from build123d import *

# Parameters (mm, degrees)
SKETCH1_W           = 190
SKETCH1_H           = 190
BOSS_EXTRUDE1_DEPTH = 5
SKETCH2_W           = 166
SKETCH2_H           = 166
CUT_EXTRUDE1_DEPTH  = 135.443296597
FILLET1_R           = 20
SKETCH3_R           = 3.05
CUT_EXTRUDE2_DEPTH  = 135.443296597
CHAMFER1_SIZE       = 10


with BuildPart() as part:
    # Sketch1 → Boss-Extrude1 (new body)
    with BuildSketch(Plane(origin=(0, 0, 0), x_dir=(1, 0, 0), z_dir=(0, 1, 0))):
        Rectangle(SKETCH1_W, SKETCH1_H)
    extrude(amount=BOSS_EXTRUDE1_DEPTH)

    # Sketch2 → Cut-Extrude1 (cut, through all)
    with BuildSketch(Plane(origin=(0, 5, 0), x_dir=(1, 0, 0), z_dir=(0, 1, 0))):
        Rectangle(SKETCH2_W, SKETCH2_H)
    extrude(amount=-CUT_EXTRUDE1_DEPTH, mode=Mode.SUBTRACT)

    # Fillet1
    fillet1_edges = [part.edges().sort_by_distance(p)[0] for p in [
        (83, 2.5, -83),
        (83, 2.5, 83),
        (-83, 2.5, 83),
        (-83, 2.5, -83),
    ]]
    fillet(fillet1_edges, radius=FILLET1_R)

    # Sketch3 → Cut-Extrude2 (cut, through all)
    with BuildSketch(Plane(origin=(0, 5, 0), x_dir=(1, 0, 0), z_dir=(0, 1, 0))):
        with Locations(Location((-77, 89, 0), (0, 0, 270))):
            Circle(SKETCH3_R)
        with Locations(Location((-89, 68, 0), (0, 0, 270))):
            Circle(SKETCH3_R)
        with Locations(Location((89, 77, 0), (0, 0, 270))):
            Circle(SKETCH3_R)
        with Locations(Location((68, 89, 0), (0, 0, 270))):
            Circle(SKETCH3_R)
        with Locations(Location((77, -89, 0), (0, 0, 270))):
            Circle(SKETCH3_R)
        with Locations(Location((89, -68, 0), (0, 0, 270))):
            Circle(SKETCH3_R)
        with Locations(Location((-89, -77, 0), (0, 0, 270))):
            Circle(SKETCH3_R)
        with Locations(Location((-68, -89, 0), (0, 0, 270))):
            Circle(SKETCH3_R)
    extrude(amount=-CUT_EXTRUDE2_DEPTH, mode=Mode.SUBTRACT)

    # Chamfer1
    chamfer1_edges = [part.edges().sort_by_distance(p)[0] for p in [
        (-95, 2.5, -95),
        (-95, 2.5, 95),
        (95, 2.5, 95),
        (95, 2.5, -95),
    ]]
    chamfer(chamfer1_edges, length=CHAMFER1_SIZE)


solid = part.part
Geometry: final body of the model. Coordinates: model frame, mm. A direction names the side the tool comes from. Round coordinates to 2 decimals unless told otherwise and drop trailing zeros. Loops run counter-clockwise (first coordinate to the right, second up) from the corner with the lowest first, then second, coordinate; pieces in that order, holes last. Notation, with made-up numbers: (-29, 17) -> (9, 17) arc R25 ccw to (9, 49) -> close; hole circle Ø2 at (24, -14). An arc over 180 degrees is marked (long way). One line per question, with ' | ' between items. Start each with the question number.
1. Mould query, pull axis X, two halves, no side actions, for faces 1 (the face through (90, 2, 90)), 2 (the face through (-86, 0, -1)), 3 (the face through (-95, 2, 1)), 4 (the face through (-88.866, 2.535, 73.953)). Classes: pulls with the +X half, pulls with the -X half, needs draft (parallel to the pull), parting line crosses it, or undercut.
2. Line query: line 1 along X through (y, z) = (3.05, -52); line 2 along X through (y, z) = (1.7, 68); line 3 along X through (y, z) = (2.25, 89). Output: solid intervals per line, ascending. Write a range as [from, to].
3. Section A-A on z = 49. Output: boundary loops of the cut face in (x, y), and give its area (3 significant figures).
4. Section D-D on y = 1.85. Count the separate pieces of the cut face and the enclosed holes in it, and give its area (3 significant figures).
5. Section C-C on x = 89. Output: boundary loops of the cut face in (y, z).
6. Section B-B on x = -48. Output: boundary loops of the cut face in (y, z), and give its area (3 significant figures).
7. Set-up query: faces 5 (the face through (-83, 3, 1)), 6 (the face through (95, 2, 1)). Return all of +Z, -Z, +X, -X, +Y, -Y with unobstructed straight access to the full face (end or side cutting, diameter ignored); none if empty.
8. Contact query for a flat-ended pin moving along its axis: pin 1 (3.5 mm diameter, centred on x = 89, z = -77, fed in from +Y). Output: stop coordinate, or through.
Returned:
1) face 1: pulls with the +X half | face 2: needs draft | face 3: pulls with the -X half | face 4: undercut
2) line 1: x = [-95, -83], [83, 95] | line 2: x = [-95, -82.36], [82.36, 85.95], [92.05, 95] | line 3: x = [-91, -71.05], [-64.95, 73.95], [80.05, 91]
3) outline: (-95, 0) -> (-83, 0) -> (-83, 5) -> (-95, 5) -> close; (83, 0) -> (95, 0) -> (95, 5) -> (83, 5) -> close | area: 120 mm2
4) separate pieces: 1 | enclosed holes: 9 | area: 8,450 mm2
5) outline: (0, -91) -> (5, -91) -> (5, -80.05) -> (0, -80.05) -> close; (0, -73.95) -> (5, -73.95) -> (5, 64.95) -> (0, 64.95) -> close; (0, 71.05) -> (5, 71.05) -> (5, 91) -> (0, 91) -> close
6) outline: (0, -95) -> (5, -95) -> (5, -83) -> (0, -83) -> close; (0, 83) -> (5, 83) -> (5, 95) -> (0, 95) -> close | area: 120 mm2
7) face 5: +Y, -Y | face 6: +Z, -Z, +X, +Y, -Y
8) pin 1: passes through
